Build history of the part. All positions in model axes, mm. Round coordinates to 2 decimals unless told otherwise and drop trailing zeros. Order: outer loops, then holes, each group sorted by start corner. A loop starts at its lowest first (then second) coordinate and runs counter-clockwise, first axis right, second up. Notation, with made-up numbers: (0.5, 88) - (38.5, 88) arc R29 ccw to (38.5, 122) - close; hole circle Ø1 at (-9.75, 39). An arc over 180 degrees is marked (long way). One line per question, with ' | ' between items. Start each with the question number.
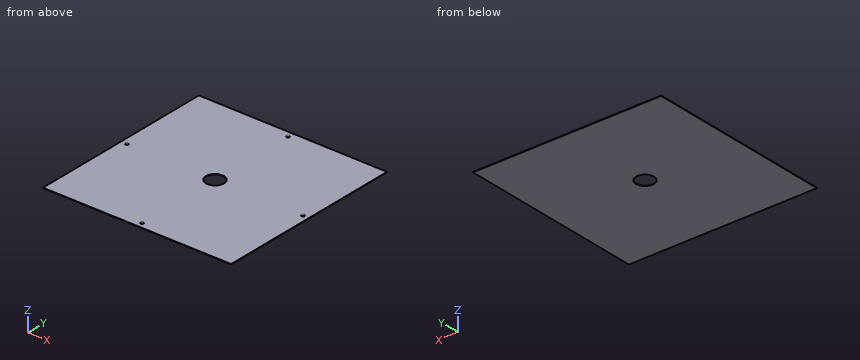
from build123d import *

# Parameters (mm, degrees)
SKETCH2_W           = 626
SKETCH2_H           = 626
SKETCH2_R           = 30
BOSS_EXTRUDE1_DEPTH = 1.5
SKETCH3_R           = 5
BOSS_EXTRUDE2_DEPTH = 1.5


with BuildPart() as part:
    # Sketch2 → Boss-Extrude1 (new body)
    with BuildSketch(Plane.XY):
        Rectangle(SKETCH2_W, SKETCH2_H)
        Circle(SKETCH2_R, mode=Mode.SUBTRACT)
    extrude(amount=BOSS_EXTRUDE1_DEPTH)

    # Sketch3 → Boss-Extrude2 (add)
    with BuildSketch(Plane.XY.offset(1.5)):
        with Locations((0, 293)):
            Circle(SKETCH3_R)
        with Locations((-293, 0)):
            Circle(SKETCH3_R)
        with Locations((0, -293)):
            Circle(SKETCH3_R)
        with Locations((293, 0)):
            Circle(SKETCH3_R)
    extrude(amount=BOSS_EXTRUDE2_DEPTH)


solid = part.part
Item 1: Slice it at B-B (x = -234). Write the cut outline in (y, z).
Item 2: Wall check: line 1 along Y through (x, z) = (0, 0.7); line 2 along Z through (x, y) = (133, -46). Give the ranges that are in metal, low to high. Write a range as [from, to].
Item 3: Slice it at A-A (y = 14). Write the cut outline in (x, z), plus the area to 3 significant figures.
A:
1) outline: (-313, 0) - (313, 0) - (313, 1.5) - (-313, 1.5) - close
2) line 1: [-313, -30], [30, 313] | line 2: [0, 1.5]
3) outline: (-313, 0) - (-26.53, 0) - (-26.53, 1.5) - (-313, 1.5) - close; (26.53, 0) - (313, 0) - (313, 1.5) - (26.53, 1.5) - close | area: 859 mm^2
